Answer from the drawing. Dimensions are ordinates in mm from the lowest x, y and z of the part. A direction names the side the tool comes from. Coordinates: 2 decimals unless noted, no trailing zeros. Order: outer loops, then holes, each group sorted by start corner. A loop starts at its lowest first (then second) coordinate and runs counter-clockwise, first axis right, second up. Notation, with made-up numbers: M 44.5,5 L 67.5,5 A18 ccw 67.5,35 Z; hole C 86,7 d11. An arc over 180 degrees is marked long. Use a Markdown table: item, result.
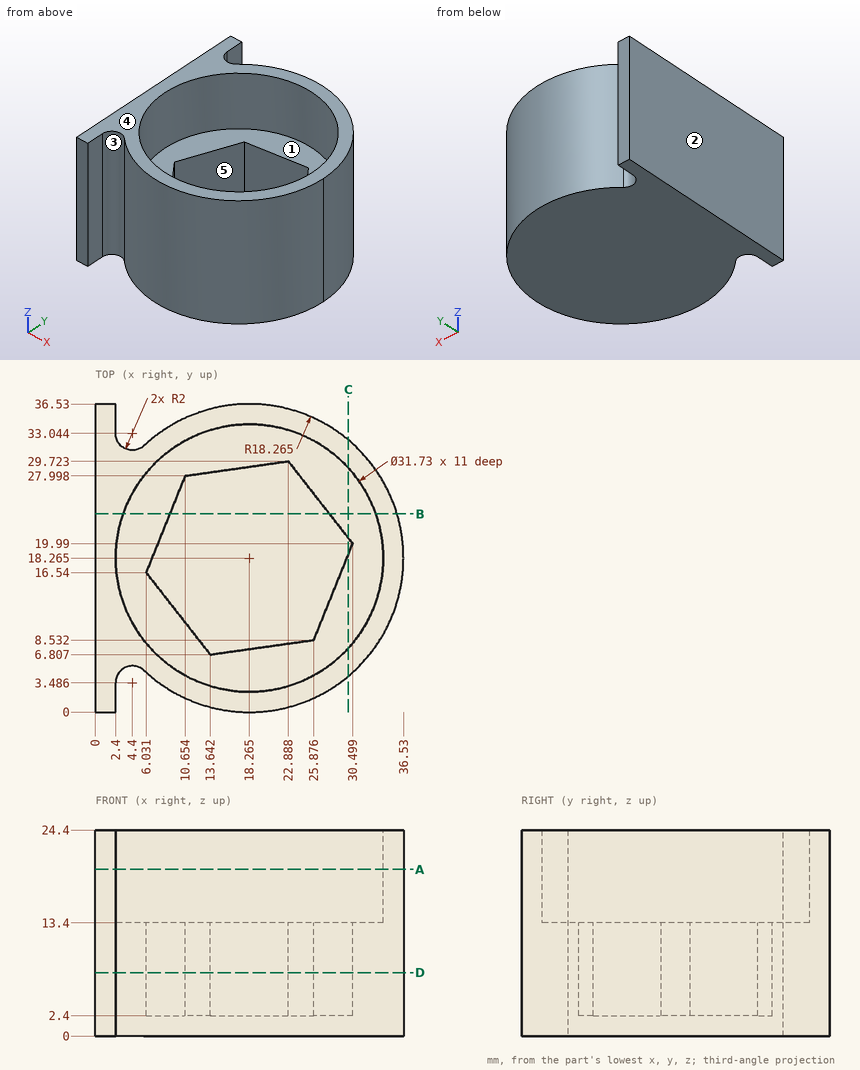
(1) A cutting plane is placed at D-D (z = 7.5). Determine the outline of the cut face in (x, y) (1 decimal).
Conclusion:
| item | result |
|---|---|
| outline | M 0,0 L 2.4,0 L 2.4,3.5 A2 cw 5.8,4.9 A18.3 ccw long 5.8,31.6 A2 cw 2.4,33 L 2.4,36.5 L 0,36.5 Z; hole M 6,16.5 L 13.6,6.8 L 25.9,8.5 L 30.5,20 L 22.9,29.7 L 10.7,28 Z |
(2) Straight lines are drawn through the part: L1, parallel to Z at x = 20.5, y = 22.5; L2, parallel to Z at x = 6, y = 13.5; L3, parallel to Y at x = 22, z = 20.75 (1 decimal). For each, find the intervals that lie inside material, in ascending order.
Conclusion:
| item | result |
|---|---|
| L1 | 0 to 2.4 |
| L2 | 0 to 13.4 |
| L3 | 0.4 to 2.8, 33.7 to 36.1 |
(3) A cutting plane is placed at C-C (x = 30). Determine the outline of the cut face in (y, z).
Conclusion:
| item | result |
|---|---|
| outline | M 4.27,0 L 32.26,0 L 32.26,24.4 L 28.94,24.4 L 28.94,13.4 L 20.63,13.4 L 20.63,2.4 L 18.75,2.4 L 18.75,13.4 L 7.59,13.4 L 7.59,24.4 L 4.27,24.4 Z |
(4) A cutting plane is placed at B-B (y = 23.5). Determine the outline of the cut face in (x, z) (1 decimal), then the cut area to 3 significant figures.
Conclusion:
| item | result |
|---|---|
| outline | M 0,0 L 35.8,0 L 35.8,24.4 L 33.2,24.4 L 33.2,13.4 L 27.8,13.4 L 27.8,2.4 L 8.8,2.4 L 8.8,13.4 L 3.3,13.4 L 3.3,24.4 L 0,24.4 Z |
| area | 335 mm2 |
(5) Given P1, Ø1, axis at y = 21, z = 20, coming from the +X side; P2, Ø1, axis at y = 2, z = 7, coming from the +X side; P3, Ø2, axis at x = 6.5, z = 20, coming from the -Y side; P4, Ø4, axis at x = 8.5, y = 32.5, coming from the -Z side, each flat-ended and moving along its own axis, determine where each tip first touches the part or whether it passes through.
Conclusion:
| item | result |
|---|---|
| P1 | x = 36.39 |
| P2 | x = 27.49 |
| P3 | y = 3.51 |
| P4 | z = 0 |
(6) A cutting plane is placed at A-A (z = 19.75). Determine the outline of the cut face in (x, y) (1 decimal).
Conclusion:
| item | result |
|---|---|
| outline | M 0,0 L 2.4,0 L 2.4,3.5 A2 cw 5.8,4.9 A18.3 ccw long 5.8,31.6 A2 cw 2.4,33 L 2.4,36.5 L 0,36.5 Z; hole C 18.3,18.3 d31.7 |
(7) Determine the mould class of the marked faces 1, 2 and 3 for opening direction Y: pulls with the +Y half, pulls with the -Y half, needs draft (parallel to the pull), parting line crosses it, or undercut.
Conclusion:
| item | result |
|---|---|
| face 1 | undercut |
| face 2 | needs draft |
| face 3 | pulls with the -Y half |
(8) Which of the six approach directions +Z, -Z, +X, -X, +Y, -Y give full straight-line access (tool end or side, diameter ignored) to the marked faces 4 and 5?
Conclusion:
| item | result |
|---|---|
| face 4 | +Z, +X, -X, +Y, -Y |
| face 5 | +Z |
